Autodesk Inventor part; units mm, degrees
ref_plane "YZ Plane" through (0, 0, 0) normal (1, 0, 0) x (0, 1, 0)
ref_plane "XZ Plane" through (0, 0, 0) normal (0, 1, 0) x (-1, 0, 0)
ref_plane "XY Plane" through (0, 0, 0) normal (0, 0, 1) x (1, 0, 0)
sketch "Sketch1" plane through (0, 0, 0) normal (0, 0, 1) x (1, 0, 0)
  line L0 (19.688, 83.3096) -> (95.888, 83.3096)
  line L1 (95.888, 83.3096) -> (95.888, 7.1096)
  line L2 (95.888, 7.1096) -> (19.688, 7.1096)
  line L3 (19.688, 7.1096) -> (19.688, 83.3096)
  circle A0 centre (57.788, 45.2096) radius 23.0341
  point P0 (0, 0)
  dimension "d0" = 76.2
  dimension "d1" = 76.2
extrude "Extrusion1" add sketch "Sketch1" along normal blind 114.3 contours L0 L1 L2 L3 | A0
fillet "Fillet1" radius 3.175 4 edges at (19.688, 83.3096, 57.15) (95.888, 83.3096, 57.15) (95.888, 7.1096, 57.15) (19.688, 7.1096, 57.15)
sketch "Sketch2" plane through (95.888, 10.2846, 0) normal (1, 0, 0) x (0, 0, -1)
  line L0 (-83.9389, 49.2214) -> (-30.1471, 49.2214) construction
  line L1 (-30.1471, 49.2214) -> (-30.1471, 33.4582) construction
  line L2 (-30.1471, 33.4582) -> (-83.9389, 33.4582) construction
  line L3 (-83.9389, 33.4582) -> (-83.9389, 49.2214) construction
  point P0 (0, -10.2846)
sketch "Sketch3" plane through (0, 0, 0) normal (0, 0, -1) x (-1, 0, 0)
  circle A0 centre (-57.788, 45.2096) radius 18.2832
  line L0 (-92.713, 7.1096) -> (-22.863, 7.1096)
  line L1 (-95.888, 80.1346) -> (-95.888, 10.2846)
  point P0 (0, 0)
  dimension "d5" = 38.1
  dimension "d6" = 38.1
extrude "Extrusion2" cut sketch "Sketch3" against normal blind 7.62
properties part number "orca flash"
Check sheet for the modelled part. Datum: model origin and axes. Units: mm. A direction names the side the tool comes from. Round coordinates to 2 decimals unless told otherwise and drop trailing zeros. Loops run counter-clockwise (first coordinate to the right, second up) from the corner with the lowest first, then second, coordinate; pieces in that order, holes last. Notation, with made-up numbers: (26.5, 43) -> (76.5, 43) arc R12 ccw to (76.5, 58) -> close; hole circle Ø5 at (59.5, -34). An arc over 180 degrees is marked (long way). Answer in a Markdown table with one row per item.
Q1. Go/stop test with a flat-tipped pin: P1, Ø18.5, axis at x = 54, y = 41.5, coming from the -Z side. Record where the tip stops, or that it passes through.
Data:
| item | result |
|---|---|
| P1 | stops at z = 7.62 |
Q2. Sectioned sample at B-B on x = 70.5. Enter the section's corners in (y, z).
Data:
| item | result |
|---|---|
| outline | (7.11, 0) -> (32.07, 0) -> (32.07, 7.62) -> (58.35, 7.62) -> (58.35, 0) -> (83.31, 0) -> (83.31, 114.3) -> (7.11, 114.3) -> close |
Q3. Thickness scan on L1, parallel to Z at x = 59.5, y = 47.5. Record the ranges inside material, lowest first.
Data:
| item | result |
|---|---|
| L1 | z = 7.62 to 114.3 |
Q4. Sectioned sample at A-A on y = 49. Enter the section's corners in (x, z), then the cut area to 3 significant figures.
Data:
| item | result |
|---|---|
| outline | (19.69, 0) -> (39.9, 0) -> (39.9, 7.62) -> (75.67, 7.62) -> (75.67, 0) -> (95.89, 0) -> (95.89, 114.3) -> (19.69, 114.3) -> close |
| area | 8,440 mm^2 |
Q5. Release check for a two-part mould opening along X. For faces 3 (the face through (58, 45, 7.62)), 4 (the face through (94.983, 82.355, 57.95)), 5 (the face through (57, 83.31, 56)) record: released by +X, released by -X, zero draft, split by the parting line, or undercut.
Data:
| item | result |
|---|---|
| face 3 | undercut |
| face 4 | released by +X |
| face 5 | zero draft |
Q6. Set-up check for faces 1 (the face through (76.054, 46.013, 3.757)), 2 (the face through (57, 46, 114.3)): record each of +Z, -Z, +X, -X, +Y, -Y from which the full face is reachable in a straight line by a thin tool's end or side.
Data:
| item | result |
|---|---|
| face 1 | -Z |
| face 2 | +Z, +X, -X, +Y, -Y |
